Autodesk Inventor part; units mm, degrees
ref_plane "YZ Plane" through (0, 0, 0) normal (1, 0, 0) x (0, 1, 0)
ref_plane "XZ Plane" through (0, 0, 0) normal (0, 1, 0) x (-1, 0, 0)
ref_plane "XY Plane" through (0, 0, 0) normal (0, 0, 1) x (1, 0, 0)
sketch "Sketch1" plane through (0, 0, 0) normal (0, 0, 1) x (1, 0, 0)
  circle A0 centre (0, 0) radius 15
  dimension "d0" = 30
extrude "Extrusion1" add sketch "Sketch1" along normal blind 40
sketch "Sketch2" plane through (0, 0, 40) normal (0, 0, 1) x (1, 0, 0)
  line L0 (7.5, 7.5) -> (7.5, -7.5)
  line L1 (-7.5, 7.5) -> (-7.5, -7.5)
  line L2 (-7.5, 7.5) -> (7.5, 7.5)
  line L3 (-7.5, -7.5) -> (7.5, -7.5)
  point P0 (0, 0)
  dimension "d3" = 7.5
  dimension "d4" = 7.5
  dimension "d5" = 7.5
  dimension "d6" = 7.5
extrude "Extrusion2" add sketch "Sketch2" along normal blind 22.5
fillet "Fillet1" radius 7.5 2 edges at (0, 7.5, 62.5) (0, -7.5, 62.5)
sketch "Sketch3" plane through (0, 0, 0) normal (1, 0, 0) x (0, 1, 0)
  line L0 (7.5, 40) -> (7.5, 55)
  line L1 (-7.5, 40) -> (-7.5, 55)
  line L2 (7.5, 55) -> (-7.5, 55) construction
  circle A0 centre (0, 55) radius 3.75
  point P0 (0, 0)
  dimension "d10" = 7.5
extrude "Extrusion3" cut sketch "Sketch3" along normal through all both and the other way through all
sketch "Sketch4" plane through (0, 0, 0) normal (0, 0, -1) x (-1, 0, 0)
  line L0 (-7.5, 7.5) -> (7.5, 7.5)
  line L1 (7.5, 7.5) -> (7.5, -7.5)
  line L2 (7.5, -7.5) -> (-7.5, -7.5)
  line L3 (-7.5, -7.5) -> (-7.5, 7.5)
  line L4 (-7.5, 7.5) -> (7.5, -7.5) construction
  line L5 (7.5, 7.5) -> (-7.5, -7.5) construction
  point P0 (0, 0)
  dimension "d13" = 15
  dimension "d14" = 15
extrude "Extrusion4" add sketch "Sketch4" along normal blind 22.5
fillet "Fillet2" radius 7.5 2 edges at (0, 7.5, -22.5) (0, -7.5, -22.5)
sketch "Sketch5" plane through (7.5, -7.5, 0) normal (1, 0, 0) x (0, 0, -1)
  line L0 (0, 15) -> (15, 15)
  line L1 (0, 0) -> (15, 0)
  line L2 (15, 15) -> (15, 0) construction
  circle A0 centre (15, 7.5) radius 3.75
  point P0 (0, 7.5)
  dimension "d18" = 7.5
extrude "Extrusion5" cut sketch "Sketch5" against normal through all
properties part number "Neck"
Here's how the part is built. I have some questions about the finished solid (model axes, mm). A direction names the side the tool comes from. Give positions to 0.01 mm unless a question says otherwise; leave off trailing zeros. Order: outer loops, then holes, each group sorted by start corner. A loop starts at its lowest first (then second) coordinate and runs counter-clockwise, first axis right, second up. Notation, with made-up numbers: (14.25, -10) -> (45.25, -10) arc R21 cw to (45.25, 16) -> close; hole circle Ø2 at (57.5, 35.5). An arc over 180 degrees is marked (long way). Use a Markdown table: item, result. Add a question column.
Item 1: If we mould it in two halves opening along Z, with no side actions, what happens to faces 5 (the face through (0.105, -5.245, 60.361)), 6 (the face through (0.11, -0.81, 51.34)), 7 (the face through (-7.5, 0, -9))? For each: pulls with the +Z half, pulls with the -Z half, needs draft (parallel to the pull), parting line crosses it, or undercut.
Item 2: Will these pins go through, and if not, where does the flat tip stop? pin 1 (16.5 mm diameter, centred on y = 1, z = 55, fed in from -X); pin 2 (12 mm diameter, centred on x = -3.5, z = 50, fed in from +Y); pin 3 (4.5 mm diameter, centred on x = 3.5, z = 49.5, fed in from -Y); pin 4 (4 mm diameter, centred on y = 10.5, z = 53.5, fed in from -X).
Item 3: Imagine slicing it at B-B on y = -1. Please give me the cut outline in (x, z).
Item 4: For faces 1 (the face through (7.5, 0, 49)), 2 (the face through (0, 7.5, -7)), 3 (the face through (7.5, 0, -9)), 4 (the face through (0, 7.5, 47)), which set-ups out of +Z, -Z, +X, -X, +Y, -Y let a thin tool reach every point of the face, with its end or its side?
Item 5: Imagine slicing it at A-A on x = 0. Give the number of separate pieces and of enclosed holes in the cut face, plus the area to 3 significant figures.
Item 6: Imagine slicing it at C-C on z = 32.5. Please give me the cut outline in (x, y), plus the area to 3 significant figures.
Item 7: I need wall thicknesses on line 1 (Z direction, x = 6.5, y = -10.25); line 2 (Y direction, x = 4.25, z = 55); line 3 (X direction, y = -5.5, z = -17.5). Which ranges of each line are inside material? Lowest first, please.
Item 8: Imagine slicing it at D-D on y = 5.5. Please give me the cut outline in (x, z), plus the area to 3 significant figures.
Data:
| question | item | result |
|---|---|---|
| 1 | face 5 | pulls with the +Z half |
| 1 | face 6 | undercut |
| 1 | face 7 | needs draft |
| 2 | pin 1 | stops at x = -7.5 |
| 2 | pin 2 | stops at y = 7.5 |
| 2 | pin 3 | stops at y = -7.5 |
| 2 | pin 4 | passes through |
| 3 | outline | (-14.97, 0) -> (-7.5, 0) -> (-7.5, -11.39) -> (7.5, -11.39) -> (7.5, 0) -> (14.97, 0) -> (14.97, 40) -> (7.5, 40) -> (7.5, 51.39) -> (-7.5, 51.39) -> (-7.5, 40) -> (-14.97, 40) -> close; (-7.5, -22.43) -> (7.5, -22.43) -> (7.5, -18.61) -> (-7.5, -18.61) -> close; (-7.5, 58.61) -> (7.5, 58.61) -> (7.5, 62.43) -> (-7.5, 62.43) -> close |
| 4 | face 1 | +Z, +X, +Y, -Y |
| 4 | face 2 | -Z, +X, -X, +Y |
| 4 | face 3 | -Z, +X, +Y, -Y |
| 4 | face 4 | +Z, +X, -X, +Y |
| 5 | separate pieces | 1 |
| 5 | enclosed holes | 2 |
| 5 | area | 1,740 mm² |
| 6 | outline | circle Ø30 at (0, 0) |
| 6 | area | 707 mm² |
| 7 | line 1 | z = 0 to 40 |
| 7 | line 2 | y = -7.5 to -3.75, 3.75 to 7.5 |
| 7 | line 3 | x = -7.5 to 7.5 |
| 8 | outline | (-13.96, 0) -> (-7.5, 0) -> (-7.5, -20.1) -> (7.5, -20.1) -> (7.5, 0) -> (13.96, 0) -> (13.96, 40) -> (7.5, 40) -> (7.5, 60.1) -> (-7.5, 60.1) -> (-7.5, 40) -> (-13.96, 40) -> close |
| 8 | area | 1,720 mm² |
